Read the model definition and answer for the solid it produces. Units are mm, in the model's axes. A direction names the side the tool comes from. Round coordinates to 2 decimals unless told otherwise and drop trailing zeros. Write each loop counter-clockwise with the first axis right and the second up, starting at its lowest first coordinate (ties: lowest second). Pieces come first, ordered by that corner, then holes.
Autodesk Fusion 360 part; units mm, degrees
sketch "Center" plane through (0, 0, 0) normal (1, 0, 0) x (0, 1, 0)
  circle A0 centre (0, 0) radius 2.7
  dimension "d1" = 5.4
extrude "Center width" add sketch "Center" along normal blind 19 makes body 1
sketch "Axis" plane through (19, 0, 0) normal (1, 0, 0) x (0, 1, 0)
  circle A0 centre (0, 0) radius 2.7
  line L0 (-1.85, 1.9666) -> (1.85, 1.9666)
  line L1 (1.85, -1.9666) -> (-1.85, -1.9666)
  arc A1 (-1.85, 1.9666) -> (-1.85, -1.9666) centre (0, 0) ccw
  arc A2 (1.85, -1.9666) -> (1.85, 1.9666) centre (0, 0) ccw
  dimension "d4" = 5.4
  dimension "d5" = 3.7
extrude "Axis width" add sketch "Axis" along normal blind 9 separate body contours A0 L0 L1 A1 A2 makes body 2
ref_plane "WorkPlane1" through (9.5, 0, 0) normal (1, 0, 0) x (0, 1, 0)
mirror "Axis mirror" about plane through (9.5, 0, 0) normal (1, 0, 0) of "Axis width" makes body 3
equation "d8 = ( 19 / 2 ) * 1 mm"

Autodesk Fusion 360 part; units mm, degrees
sketch "Motor base" plane through (0, 0, 0) normal (0, 0, 1) x (1, 0, 0)
  line L0 (0, 0) -> (0, -16)
  line L1 (0, -8) -> (-19, -8) construction
  line L2 (-9.5, -8) -> (-9.5, -19) construction
  line L3 (-19, 0) -> (-19, -16)
  arc A0 (-19, -16) -> (0, -16) centre (-9.5, -2.4583) ccw
  arc A1 (0, 0) -> (-19, 0) centre (-9.5, -13.5417) ccw
  dimension "d1" = 16
  dimension "d2" = 19
  dimension "d3" = 11
extrude "Motor height" add sketch "Motor base" along normal blind 17
equation "d1 = 22 mm - 6 mm"

Autodesk Fusion 360 part; units mm, degrees
sketch "Case base" plane through (0, 0, 0) normal (1, 0, 0) x (0, 1, 0)
  line L0 (-11, 24) -> (11, 24)
  line L1 (11, 24) -> (11, -21)
  line L2 (8, -24) -> (-8, -24)
  line L3 (-11, -21) -> (-11, 24)
  line L4 (-11, 24) -> (11, -24) construction
  line L5 (11, 24) -> (-11, -24) construction
  arc A0 (-11, -21) -> (-8, -24) centre (-8, -21) ccw
  arc A1 (8, -24) -> (11, -21) centre (8, -21) ccw
  dimension "d5" = 22
  dimension "d6" = 48
  dimension "d7" = 3
  dimension "d8" = 3
extrude "Case width" add sketch "Case base" along normal blind 19
sketch "Pin base" plane through (0, 0, -24) normal (0, 0, -1) x (1, 0, 0)
  line L0 (0, 8) -> (0, -8)
  line L1 (0, -8) -> (19, -8)
  line L2 (19, -8) -> (19, 8)
  line L3 (19, 8) -> (0, 8)
  line L4 (0, 0) -> (19, 0) construction
  line L5 (11, 2.5) -> (8, 2.5)
  line L6 (8, 2.5) -> (8, -2.5)
  line L7 (8, -2.5) -> (11, -2.5)
  line L8 (11, -2.5) -> (11, 2.5)
  line L9 (11, 2.5) -> (8, -2.5) construction
  line L10 (8, 2.5) -> (11, -2.5) construction
  point P0 (9.5, 0)
  dimension "d11" = 5
  dimension "d12" = 3
extrude "Pin base (1)" add sketch "Pin base" along normal blind 5 contours L5 L6 L7 L8
sketch "Pin hole" plane through (11, 0, 0) normal (1, 0, 0) x (0, 1, 0)
  line L0 (2.5, -24) -> (-2.5, -24)
  line L1 (-2.5, -24) -> (-2.5, -29)
  line L2 (-2.5, -29) -> (2.5, -29)
  line L3 (2.5, -29) -> (2.5, -24)
  circle A0 centre (0, -26.5) radius 1.5
  dimension "d15" = 3
extrude "Pin hole (1)" cut sketch "Pin hole" along normal through all contours A0
sketch "Case axis" plane through (19, 0, 0) normal (1, 0, 0) x (0, 1, 0)
  arc A0 (-11, -21) -> (-8, -24) centre (-8, -21) ccw
  line L0 (-8, -24) -> (8, -24)
  arc A1 (8, -24) -> (11, -21) centre (8, -21) ccw
  line L1 (11, -21) -> (11, 24)
  line L2 (11, 24) -> (-11, 24)
  line L3 (-11, 24) -> (-11, -21)
  line L4 (0, -24) -> (0, -12) construction
  circle A2 centre (0, -12) radius 2.7
  dimension "d17" = 12
  dimension "d18" = 5.4
extrude "Case axis (1)" cut sketch "Case axis" against normal through all contours A2
sketch "Case hole" plane through (19, 0, 0) normal (1, 0, 0) x (0, 1, 0)
  circle A0 centre (0, -12) radius 2.7
  arc A1 (-11, -21) -> (-8, -24) centre (-8, -21) ccw
  line L0 (-8, -24) -> (8, -24)
  arc A2 (8, -24) -> (11, -21) centre (8, -21) ccw
  line L1 (11, -21) -> (11, 24)
  line L2 (11, 24) -> (-11, 24)
  line L3 (-11, 24) -> (-11, -21)
  line L4 (-11, 22) -> (-9, 22) construction
  line L5 (-9, 24) -> (-9, 7) construction
  circle A3 centre (-9, 7) radius 1.5
  dimension "d20" = 2
  dimension "d21" = 17
  dimension "d22" = 3
extrude "Case hole (1)" cut sketch "Case hole" against normal through all contours A3
mirror "Case holes" about plane through (0, 0, 0) normal (0, 1, 0) of "Case hole (1)"
Q1. Section A-A (z = -12) is taken. Determine the outline of the cut face in (x, y), then the cut area to 3 significant figures.
Verdict:
outline: (0, -11) - (19, -11) - (19, -2.7) - (0, -2.7) - close; (0, 2.7) - (19, 2.7) - (19, 11) - (0, 11) - close
area: 315 mm2
Q2. Section C-C (x = 15) is taken. Determine the outline of the cut face in (y, z), then the cut area to 3 significant figures.
Verdict:
outline: (-11, -21) arc R3 ccw to (-8, -24) - (8, -24) arc R3 ccw to (11, -21) - (11, 24) - (-11, 24) - close; hole circle Ø3 at (-9, 7); hole circle Ø5.4 at (0, -12); hole circle Ø3 at (9, 7)
area: 1,020 mm2
Q3. Section D-D (y = -9) is taken. Determine the outline of the cut face in (x, z), then the cut area to 3 significant figures.
Verdict:
outline: (-19, 0) - (0, 0) - (0, -23.83) - (19, -23.83) - (19, 5.5) - (-19, 5.5) - close; (-19, 8.5) - (19, 8.5) - (19, 24) - (0, 24) - (0, 17) - (-19, 17) - close
area: 1,120 mm2
Q4. Flat-ended cylindrical pins translate along their axes: pin 1 Ø5 at (y, z) = (-9, 7) entering from +X; pin 2 Ø2.5 at (x, z) = (9.5, -25.5) entering from -Y; pin 3 Ø5.5 at (y, z) = (1, -26) entering from -X; pin 4 Ø8 at (x, y) = (6.5, 6) entering from -Z. Find the tip coordinate at first contact, or state that the pin passes through.
Verdict:
pin 1: stops at x = 19
pin 2: stops at y = -2.5
pin 3: stops at x = 0
pin 4: stops at z = -29
Q5. Which of the six approach directions +Z, -Z, +X, -X, +Y, -Y give full straight-line access (tool end or side, diameter ignored) to faces 5 (the flat face through (10, -2.5, -26)), 6 (the cylindrical face through (23.4, -2.7, 0)), 7 (the flat face through (23, 0, -1.967)), 8 (the flat face through (0, -13, 8)), 9 (the flat face through (-9, 0, -1))?
Verdict:
face 5: -Z, +X, -X, -Y
face 6: +X, -Y
face 7: -Z, +X, +Y, -Y
face 8: +Z, -Z, +X, -Y
face 9: -Z, -X, +Y, -Y
Q6. Determine the mould class of faces 1 (the flat face through (8, 0, -26)), 2 (the flat face through (-10, -8, 17)), 3 (the flat face through (-1, 1, 1.967)), 4 (the flat face through (28, 0, 0)) for opening direction X: pulls with the +X half, pulls with the -X half, needs draft (parallel to the pull), parting line crosses it, or undercut.
Verdict:
face 1: pulls with the -X half
face 2: needs draft
face 3: undercut
face 4: pulls with the +X half
Q7. Straight lines are drawn through the part: probe 1 along Z at (x, y) = (-4, -11); probe 2 along X at (y, z) = (-3, -1); probe 3 along X at (y, z) = (2.25, -26). For each, find the intervals that lie inside material, in ascending order.
Verdict:
probe 1: z = 0 to 17
probe 2: x = 0 to 19
probe 3: x = 8 to 11
Q8. Section B-B (z = 7) is taken. Determine the outline of the cut face in (x, y).
Verdict:
outline: (-19, -16) arc R16.54 ccw to (0, -16) - (0, -11) - (19, -11) - (19, -10.5) - (-19, -10.5) - close; (-19, -7.5) - (19, -7.5) - (19, 7.5) - (0, 7.5) - (0, 0) arc R16.54 ccw to (-19, 0) - close; (0, 10.5) - (19, 10.5) - (19, 11) - (0, 11) - close
